The listing builds one solid part. Answer for the finished solid, in the listing's coordinates (mm). Face numbers are marked on the shaded views. A direction names the side the tool comes from. Give positions to 0.01 mm unless a question says otherwise; leave off trailing zeros. Loops run counter-clockwise (first coordinate to the right, second up) from the corner with the lowest first, then second, coordinate; pieces in that order, holes last.
Item 1: Consider line 1 along Z through (x, y) = (-11, 41.5); line 2 along X through (y, z) = (38.5, 10); line 3 along Y through (x, z) = (4, -19). Determine where each line is inside the solid, lowest interval first.
Item 2: A tool of negligible diameter and unlimited length cuts with its end or side. For the marked faces 1 and 2, from which of +Z, -Z, +X, -X, +Y, -Y can it reach the whole face along a straight path? Write none if from no direction.
Item 3: Section C-C, the plane y = -16.5 is taken. Give the vertices of the cut face in (x, z).
Item 4: Section B-B, the plane z = 0 is taken. Give the vertices of the cut face in (x, y), and give its area (3 significant figures).
Item 5: Section A-A, the plane x = 0 is taken. Give the vertices of the cut face in (y, z).
Item 6: Each of these flat-tipped pins is pushed along its axis until it touches: pin 1 Ø4 at (x, z) = (-9.9, 9.9) entering from +Y; pin 2 Ø6 at (y, z) = (26, 14.5) entering from +X; pin 3 Ø8 at (x, z) = (13.5, 3.5) entering from +Y. Where does it stop, or does it pass through?
Item 7: Section D-D, the plane x = 12.5 is taken. Give the vertices of the cut face in (y, z), and give its area (3 significant figures).
from build123d import *

# Parameters (mm, degrees)
ESQUISSE1_W                  = 42.3
ESQUISSE1_H                  = 42.3
MOTEUR_DEPTH                 = 48
CHANFREIN1_SIZE              = 4
ESQUISSE2_R                  = 18
BOSS_EXTRU_2_DEPTH           = 42.7
ESQUISSE3_R                  = 11
BOSS_EXTRU_3_DEPTH           = 2
ESQUISSE4_R                  = 4
BOSS_EXTRU_4_DEPTH           = 18
ESQUISSE5_W                  = 5.291502622
ESQUISSE5_H                  = 1
ENL_V_MAT_EXTRU_1_DEPTH      = 15
R_P_TITION_CIRCULAIRE1_COUNT = 4


with BuildPart() as part:
    # Esquisse1 → Moteur (new body)
    with BuildSketch(Plane(origin=(0, 0, 0), x_dir=(1, 0, 0), z_dir=(0, 1, 0))):
        Rectangle(ESQUISSE1_W, ESQUISSE1_H)
    extrude(amount=-MOTEUR_DEPTH)

    # Chanfrein1
    chanfrein1_edges = [part.edges().sort_by_distance(p)[0] for p in [
        (-21.15, -24, -21.15),
        (21.15, -24, -21.15),
        (21.15, -24, 21.15),
        (-21.15, -24, 21.15),
    ]]
    chamfer(chanfrein1_edges, length=CHANFREIN1_SIZE)

    # Esquisse2 → Boss.-Extru.2 (add)
    with BuildSketch(Plane(origin=(0, 0, 0), x_dir=(1, 0, 0), z_dir=(0, 1, 0))):
        with Locations(Location((0, 0, 0), (0, 0, 90))):
            Circle(ESQUISSE2_R)
    extrude(amount=BOSS_EXTRU_2_DEPTH)

    # Esquisse3 → Boss.-Extru.3 (add)
    with BuildSketch(Plane(origin=(0, 42.7, 0), x_dir=(1, 0, 0), z_dir=(0, 1, 0))):
        with Locations(Location((0, 0, 0), (0, 0, 270))):
            Circle(ESQUISSE3_R)
    extrude(amount=BOSS_EXTRU_3_DEPTH)

    # Esquisse4 → Boss.-Extru.4 (add)
    with BuildSketch(Plane(origin=(0, 44.7, 0), x_dir=(1, 0, 0), z_dir=(0, 1, 0))):
        with Locations(Location((0, 0, 0), (0, 0, 270))):
            Circle(ESQUISSE4_R)
    extrude(amount=BOSS_EXTRU_4_DEPTH)

    # Esquisse5 → Enl_v. mat.-Extru.1 (cut)
    with BuildSketch(Plane(origin=(0, 62.7, 0), x_dir=(1, 0, 0), z_dir=(0, 1, 0))):
        with Locations((0, 3.5)):
            Rectangle(ESQUISSE5_W, ESQUISSE5_H)
    extrude(amount=-ENL_V_MAT_EXTRU_1_DEPTH, mode=Mode.SUBTRACT)

    # Esquisse7 → Trou pour taraudage pour trou taraud_ M3 (revolve, cut)
    with BuildSketch(Plane(origin=(-9.899494937, 42.7, -9.899494937), x_dir=(0, 0, 1), z_dir=(1, 0, 0))):
        Polygon((0, 0), (0, 5.751075774), (1.25, 5), (1.25, 0), align=None)
    trou_pour_taraudage_pour_trou_taraud_m3 = revolve(axis=Axis((-9.899494937, 49.05, -9.899494937), (0, -1, 0)), mode=Mode.SUBTRACT)

    # R_p_tition circulaire1: Trou pour taraudage pour trou taraud_ M3 ×4 about axis
    r_p_tition_circulaire1_axis = Axis((0, 0, 0), (0, 1, 0))
    for i in range(1, R_P_TITION_CIRCULAIRE1_COUNT):
        add(trou_pour_taraudage_pour_trou_taraud_m3.rotate(r_p_tition_circulaire1_axis, i * 360 / R_P_TITION_CIRCULAIRE1_COUNT), mode=Mode.SUBTRACT)


solid = part.part
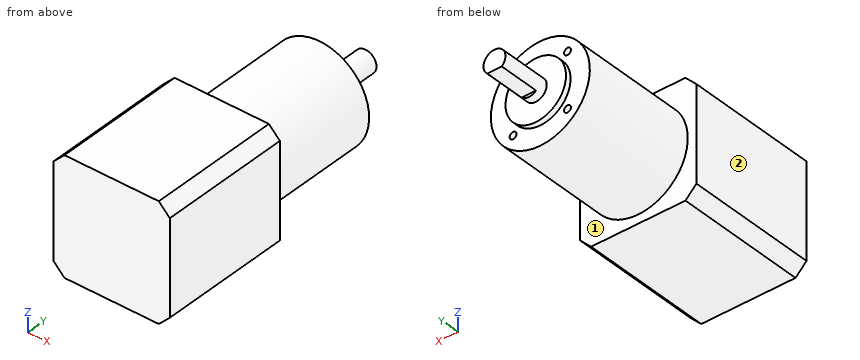
Worked answers:
1. line 1: z = -14.25 to -10.49, -9.31 to 9.31, 10.49 to 14.25
1. line 2: x = -14.97 to -11.15, -8.65 to 8.65, 11.15 to 14.97
1. line 3: y = -48 to 0
2. face 1: +Y
2. face 2: +Z, -Z, -X, +Y, -Y
3. outline: (-21.15, -17.15) - (-17.15, -21.15) - (17.15, -21.15) - (21.15, -17.15) - (21.15, 17.15) - (17.15, 21.15) - (-17.15, 21.15) - (-21.15, 17.15) - close
4. outline: (-21.15, -48) - (21.15, -48) - (21.15, 0) - (18, 0) - (18, 42.7) - (11, 42.7) - (11, 44.7) - (4, 44.7) - (4, 62.7) - (-4, 62.7) - (-4, 44.7) - (-11, 44.7) - (-11, 42.7) - (-18, 42.7) - (-18, 0) - (-21.15, 0) - close
4. area: 3,760 mm2
5. outline: (-48, -21.15) - (0, -21.15) - (0, -18) - (42.7, -18) - (42.7, -11) - (44.7, -11) - (44.7, -4) - (47.7, -4) - (47.7, -3) - (62.7, -3) - (62.7, 4) - (44.7, 4) - (44.7, 11) - (42.7, 11) - (42.7, 18) - (0, 18) - (0, 21.15) - (-48, 21.15) - close
6. pin 1: stops at y = 42.7
6. pin 2: stops at x = 13.85
6. pin 3: stops at y = 44.7
7. outline: (-48, -21.15) - (0, -21.15) - (0, -12.95) - (42.7, -12.95) - (42.7, 12.95) - (0, 12.95) - (0, 21.15) - (-48, 21.15) - close
7. area: 3,140 mm2
